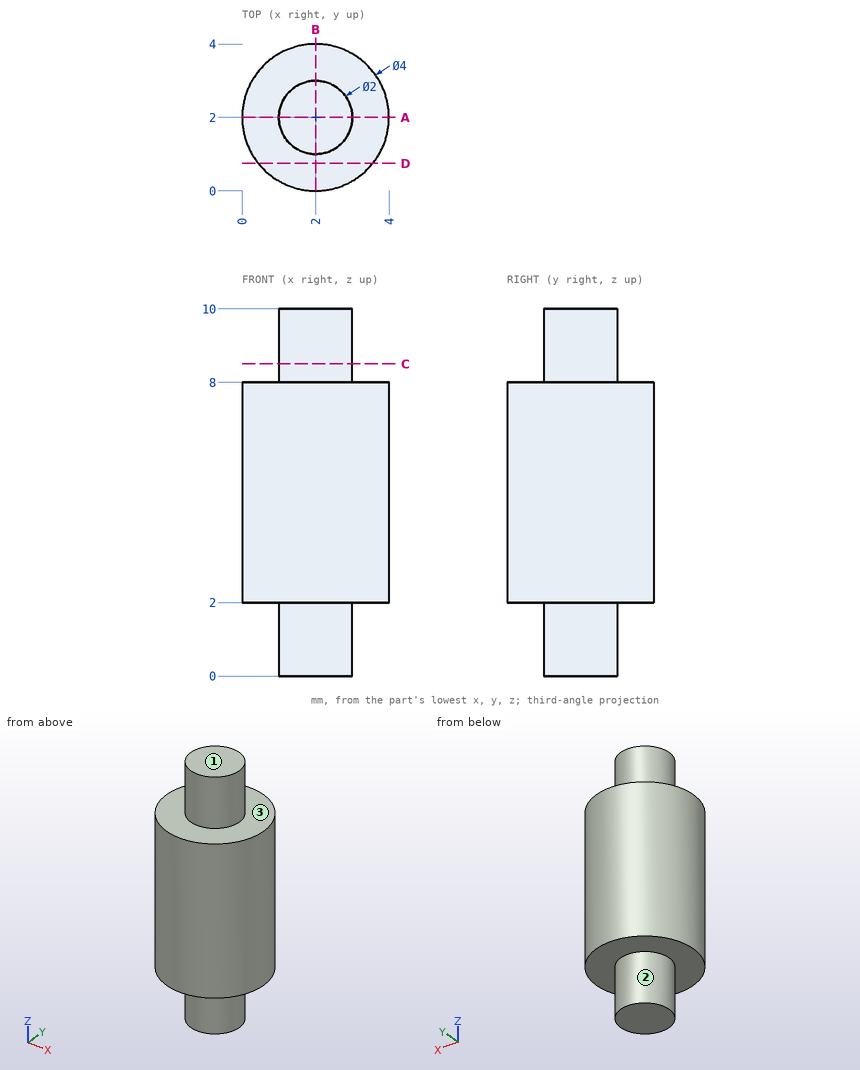
Verification items for this drawing (mm, ordinates from the low corner). A direction names the side the tool comes from. Round coordinates to 2 decimals unless told otherwise and drop trailing zeros. Write each loop counter-clockwise with the first axis right and the second up, starting at its lowest first coordinate (ties: lowest second). Pieces come first, ordered by that corner, then holes. Notation, with made-up numbers: M -31,79.5 L 22,79.5 A32 ccw 22,114.5 Z; hole C 52,72.25 d8. An arc over 180 degrees is marked long. Write item = value, one per line. Start each with the question number.
1. Section check C-C, the plane z = 8.5. Record the cut outline in (x, y), then the cut area to 3 significant figures.
2. Gauge pin test, flat ends, axial feed: pin 1 (1.5 mm diameter, centred on y = 1, z = 2.5, fed in from -X); pin 2 (1 mm diameter, centred on x = 3.5, y = 0.5, fed in from +Z). Record the tip position at first contact, or that the pin passes through.
3. Scan lines: line 1 (Z direction, x = 3.3, y = 1.45); line 2 (X direction, y = 3.7, z = 3.25); line 3 (Y direction, x = 1.65, z = 4.5). Record each from-to range of solid material in increasing order. Write a range as [from, to].
4. Section check A-A, the plane y = 2. Record the cut outline in (x, z).
5. Section check D-D, the plane y = 0.75. Record the cut outline in (x, z).
6. Tool access check on the marked faces 1, 2 and 3. Record the directions out of +Z, -Z, +X, -X, +Y, -Y that give a thin tool (end or side, any length) a straight path to the whole face; none if there is none.
Results found:
q1.outline = C 2,2 d2
q1.area = 3.14 mm^2
q2.pin_1 = 0.02
q2.pin_2 = 8
q3.line_1 = [2, 8]
q3.line_2 = [0.95, 3.05]
q3.line_3 = [0.03, 3.97]
q4.outline = M 0,2 L 1,2 L 1,0 L 3,0 L 3,2 L 4,2 L 4,8 L 3,8 L 3,10 L 1,10 L 1,8 L 0,8 Z
q5.outline = M 0.44,2 L 3.56,2 L 3.56,8 L 0.44,8 Z
q6.face_1 = +Z, +X, -X, +Y, -Y
q6.face_2 = -Z
q6.face_3 = +Z
